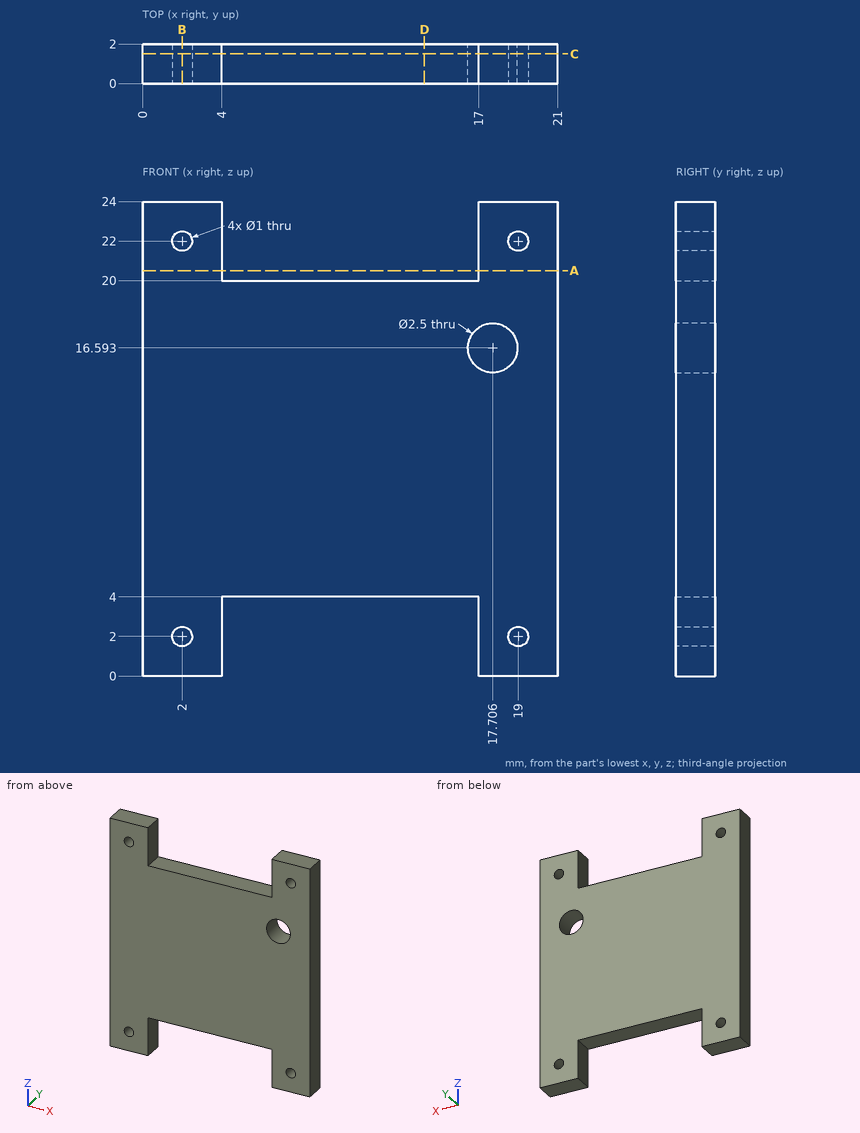
Input: dimensioned drawing with shaded views. Units: mm. Origin: part minimum x, y, z. Coordinates: 2 decimals unless noted, no trailing zeros. Write each loop counter-clockwise with the first axis right and the second up, starting at its lowest first coordinate (ties: lowest second). Pieces come first, ordered by that corner, then holes. Notation, with made-up numbers: M 48.5,-25.75 L 52.5,-25.75 A15 cw 52.5,-18.75 Z; hole C 18,-2 d6. An arc over 180 degrees is marked long. Answer as a JSON object with one key per item and string values. Group by question number.
(1) Section C-C on y = 1.5. Give the number of separate pieces and of enclosed holes in the cut face, plus the area to 3 significant figures.
(2) Section A-A on z = 20.5. Output: boundary loops of the cut face in (x, y), plus the area to 3 significant figures.
(3) Contact query for a flat-ended pin moving along its axis: P1, Ø0.6, axis at x = 8.5, y = 1.5, coming from the -Z side. Output: stop coordinate, or through.
(4) Section B-B on x = 2. Output: boundary loops of the cut face in (y, z).
(5) Section D-D on x = 14.25. Output: boundary loops of the cut face in (y, z).
(6) Ray query, line 1 along X through (y, z) = (1.5, 22.25); line 2 along X through (y, z) = (0.2, 20.75); line 3 along Z through (x, y) = (17.25, 1.2). Return the intervals inside material, ascending. Write a range as [from, to].
Result set:
{
 "1": {"separate pieces": "1", "enclosed holes": "5", "area": "392 mm2"},
 "2": {"outline": "M 0,0 L 4,0 L 4,2 L 0,2 Z; M 17,0 L 21,0 L 21,2 L 17,2 Z", "area": "16.0 mm2"},
 "3": {"P1": "stops at z = 4"},
 "4": {"outline": "M 0,0 L 2,0 L 2,1.5 L 0,1.5 Z; M 0,2.5 L 2,2.5 L 2,21.5 L 0,21.5 Z; M 0,22.5 L 2,22.5 L 2,24 L 0,24 Z"},
 "5": {"outline": "M 0,4 L 2,4 L 2,20 L 0,20 Z"},
 "6": {"line 1": "x = [0, 1.57], [2.43, 4], [17, 18.57], [19.43, 21]", "line 2": "x = [0, 4], [17, 21]", "line 3": "z = [0, 15.43], [17.76, 24]"}
}
